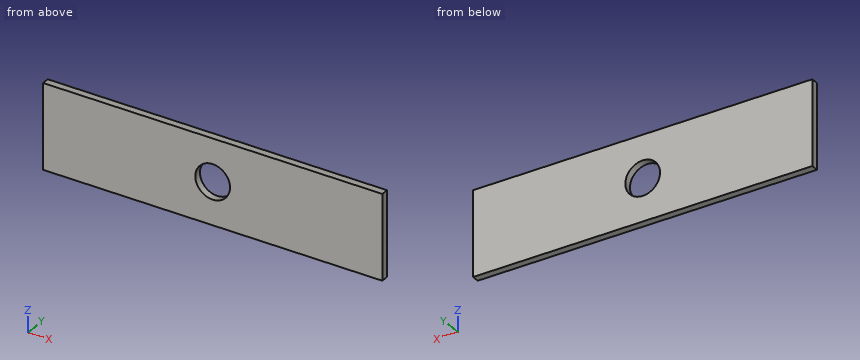
from build123d import *

# Parameters (mm, degrees)
SKETCH1_W                = 100
SKETCH1_H                = 25
BOSS_EXTRUDE1_DEPTH      = 1.075
BOSS_EXTRUDE1_DEPTH_BACK = 1.075
SKETCH2_R                = 5.12
CUT_EXTRUDE1_DEPTH       = 2.075
CUT_EXTRUDE1_DEPTH_BACK  = 2.075


with BuildPart() as part:
    # Sketch1 → Boss-Extrude1 (new body, two sides)
    with BuildSketch(Plane(origin=(0, 0, 0), x_dir=(1, 0, 0), z_dir=(0, 1, 0))) as boss_extrude1_sk:
        Rectangle(SKETCH1_W, SKETCH1_H)
    extrude(amount=BOSS_EXTRUDE1_DEPTH)
    extrude(boss_extrude1_sk.sketch, amount=-BOSS_EXTRUDE1_DEPTH_BACK)

    # Sketch2 → Cut-Extrude1 (cut, two sides)
    with BuildSketch(Plane(origin=(0, 0, 0), x_dir=(1, 0, 0), z_dir=(0, 1, 0))) as cut_extrude1_sk:
        Circle(SKETCH2_R)
    extrude(amount=CUT_EXTRUDE1_DEPTH, mode=Mode.SUBTRACT)
    extrude(cut_extrude1_sk.sketch, amount=-CUT_EXTRUDE1_DEPTH_BACK, mode=Mode.SUBTRACT)


solid = part.part
Part model, mm, in its own coordinate system. Give positions to 0.01 mm unless a question says otherwise; leave off trailing zeros. Loops run counter-clockwise (first coordinate to the right, second up) from the corner with the lowest first, then second, coordinate; pieces in that order, holes last. Notation, with made-up numbers: M 24.5,60 L 55.5,60 A11 cw 55.5,76 Z; hole C -22.5,81 d2. An arc over 180 degrees is marked long. Put each result on its own line as item: value. Start each with the question number.
1) Saw through at B-B (z = 0). List the corners of the cut face in (x, y) (3 decimals).
2) Saw through at A-A (x = 0). List the corners of the cut face in (y, z) (3 decimals).
3) Saw through at C-C (y = -0.7). List the corners of the cut face in (x, z), then the cut area to 3 significant figures.
4) Probe probe 1 along Z at (x, y) = (0, 0.5); probe 2 along X at (y, z) = (0.55, 0); probe 3 along X at (y, z) = (0.9, -3.25). List the from-to ranges inside material, lowest first.
Numbers:
1. outline: M -50,-1.075 L -5.12,-1.075 L -5.12,1.075 L -50,1.075 Z; M 5.12,-1.075 L 50,-1.075 L 50,1.075 L 5.12,1.075 Z
2. outline: M -1.075,-12.5 L 1.075,-12.5 L 1.075,-5.12 L -1.075,-5.12 Z; M -1.075,5.12 L 1.075,5.12 L 1.075,12.5 L -1.075,12.5 Z
3. outline: M -50,-12.5 L 50,-12.5 L 50,12.5 L -50,12.5 Z; hole C 0,0 d10.24
3. area: 2,420 mm^2
4. probe 1: -12.5 to -5.12, 5.12 to 12.5
4. probe 2: -50 to -5.12, 5.12 to 50
4. probe 3: -50 to -3.96, 3.96 to 50
